Could you check a few things on this model? Use its own coordinates, in mm. Face numbers are marked on the shaded views. A direction names the side the tool comes from. Give positions to 0.01 mm unless a question says otherwise; leave off trailing zeros. Order: outer loops, then holes, each group sorted by start corner. A loop starts at its lowest first (then second) coordinate and runs counter-clockwise, first axis right, second up. Notation, with made-up numbers: M 13,8.25 L 31,8.25 A22 cw 31,40.25 Z; hole C -17,28.25 d8. An arc over 180 degrees is marked long. Answer in a Markdown table with one row per item. Add a question column.
```python
from build123d import *

# Parameters (mm, degrees)
SKETCH1_W                  = 10
SKETCH1_H                  = 10
BOSS_EXTRUDE1_DEPTH        = 10
SKETCH1_3_W                = 10
SKETCH1_3_H                = 10
BOSS_EXTRUDE2_DEPTH        = 15
BOSS_EXTRUDE3_DEPTH        = 15
SKETCH3_W                  = 20
SKETCH3_H                  = 5
BOSS_EXTRUDE4_DEPTH        = 20
F_4_0_209_DIAMETER_HOLE1_D = 5.3086
SKETCH5_W                  = 193
SKETCH5_H                  = 25
BOSS_EXTRUDE5_DEPTH        = 10
F_4_0_209_DIAMETER_HOLE2_D = 5.3086


with BuildPart() as part:
    # Sketch1 → Boss-Extrude1 (new body)
    with BuildSketch(Plane(origin=(0, 0, 0), x_dir=(1, 0, 0), z_dir=(0, 1, 0))):
        with Locations((-71.5, -38)):
            Rectangle(SKETCH1_W, SKETCH1_H)
        with Locations((-71.5, -48)):
            Rectangle(SKETCH1_W, SKETCH1_H)
        with Locations((-61.5, -48)):
            Rectangle(SKETCH1_W, SKETCH1_H)
        with Locations((-71.5, 38)):
            Rectangle(SKETCH1_W, SKETCH1_H)
        with Locations((-71.5, 48)):
            Rectangle(SKETCH1_W, SKETCH1_H)
        with Locations((-61.5, 48)):
            Rectangle(SKETCH1_W, SKETCH1_H)
        with Locations((61.5, 48)):
            Rectangle(SKETCH1_W, SKETCH1_H)
        with Locations((71.5, 48)):
            Rectangle(SKETCH1_W, SKETCH1_H)
        with Locations((71.5, 38)):
            Rectangle(SKETCH1_W, SKETCH1_H)
        with Locations((61.5, -48)):
            Rectangle(SKETCH1_W, SKETCH1_H)
        with Locations((71.5, -48)):
            Rectangle(SKETCH1_W, SKETCH1_H)
        with Locations((71.5, -38)):
            Rectangle(SKETCH1_W, SKETCH1_H)
    extrude(amount=BOSS_EXTRUDE1_DEPTH)

    # Sketch1_3 → Boss-Extrude2 (add)
    with BuildSketch(Plane(origin=(0, 0, 0), x_dir=(1, 0, 0), z_dir=(0, 1, 0))):
        with Locations((-71.5, -48)):
            Rectangle(SKETCH1_3_W, SKETCH1_3_H)
        with Locations((-61.5, -38)):
            Rectangle(SKETCH1_3_W, SKETCH1_3_H)
        with Locations((-61.5, -48)):
            Rectangle(SKETCH1_3_W, SKETCH1_3_H)
        with Locations((-71.5, -38)):
            Rectangle(SKETCH1_3_W, SKETCH1_3_H)
        with Locations((71.5, -48)):
            Rectangle(SKETCH1_3_W, SKETCH1_3_H)
        with Locations((71.5, -38)):
            Rectangle(SKETCH1_3_W, SKETCH1_3_H)
        with Locations((61.5, -48)):
            Rectangle(SKETCH1_3_W, SKETCH1_3_H)
        with Locations((61.5, -38)):
            Rectangle(SKETCH1_3_W, SKETCH1_3_H)
        with Locations((71.5, 38)):
            Rectangle(SKETCH1_3_W, SKETCH1_3_H)
        with Locations((71.5, 48)):
            Rectangle(SKETCH1_3_W, SKETCH1_3_H)
        with Locations((61.5, 48)):
            Rectangle(SKETCH1_3_W, SKETCH1_3_H)
        with Locations((61.5, 38)):
            Rectangle(SKETCH1_3_W, SKETCH1_3_H)
        with Locations((-61.5, 48)):
            Rectangle(SKETCH1_3_W, SKETCH1_3_H)
        with Locations((-61.5, 38)):
            Rectangle(SKETCH1_3_W, SKETCH1_3_H)
        with Locations((-71.5, 38)):
            Rectangle(SKETCH1_3_W, SKETCH1_3_H)
        with Locations((-71.5, 48)):
            Rectangle(SKETCH1_3_W, SKETCH1_3_H)
    extrude(amount=-BOSS_EXTRUDE2_DEPTH)

    # Sketch2 → Boss-Extrude3 (add)
    with BuildSketch(Plane(origin=(0, 0, 0), x_dir=(1, 0, 0), z_dir=(0, 1, 0))):
        Polygon((-59.664368284, 52.338863371), (-72.335631716, 32.661136629), (-21.409556012, -0.132169696), (0.205251763, 13.786456523), align=None)
        Polygon((0.205251763, 13.786456523), (-21.409556012, -0.132169696), (-0.205251763, -13.786456523), (21.409556012, 0.132169696), align=None)
        Polygon((59.784693164, 52.15200591), (0.205251763, 13.786456523), (21.409556012, 0.132169696), (72.215306836, 32.84799409), align=None)
        Polygon((21.409556012, 0.132169696), (-0.205251763, -13.786456523), (59.664368284, -52.338863371), (72.335631716, -32.661136629), align=None)
        Polygon((-0.205251763, -13.786456523), (-21.409556012, -0.132169696), (-72.215306836, -32.84799409), (-59.784693164, -52.15200591), align=None)
    extrude(amount=-BOSS_EXTRUDE3_DEPTH)

    # Sketch3 → Boss-Extrude4 (add)
    with BuildSketch(Plane.ZY.offset(76.5)):
        with Locations((-43, 7.5)):
            Rectangle(SKETCH3_W, SKETCH3_H)
        with Locations((43, 7.5)):
            Rectangle(SKETCH3_W, SKETCH3_H)
    boss_extrude4 = extrude(amount=BOSS_EXTRUDE4_DEPTH)

    # Mirror1: Boss-Extrude4 across plane
    add(boss_extrude4.mirror(Plane(origin=(0, 0, 0), x_dir=(0, 0, 1), z_dir=(1, 0, 0))))

    # 4 _0.209_ Diameter Hole1 (through all)
    with Locations(Plane(origin=(-86, 10, -42.5), x_dir=(0, 0, 1), z_dir=(0, 1, 0))):
        with Locations((0, 0), (85, 0), (0, 172), (85, 172)):
            Hole(F_4_0_209_DIAMETER_HOLE1_D / 2)

    # Sketch5 → Boss-Extrude5 (add)
    with BuildSketch(Plane.XY.offset(53)):
        with Locations((0, -2.5)):
            Rectangle(SKETCH5_W, SKETCH5_H)
    extrude(amount=BOSS_EXTRUDE5_DEPTH)

    # 4 _0.209_ Diameter Hole2 (through all)
    with Locations(Plane(origin=(0, 0, 53), x_dir=(-1, 0, 0), z_dir=(0, 0, -1))):
        with Locations((-86.5, -2.674811851), (86.5, -2.5)):
            Hole(F_4_0_209_DIAMETER_HOLE2_D / 2)


solid = part.part
```
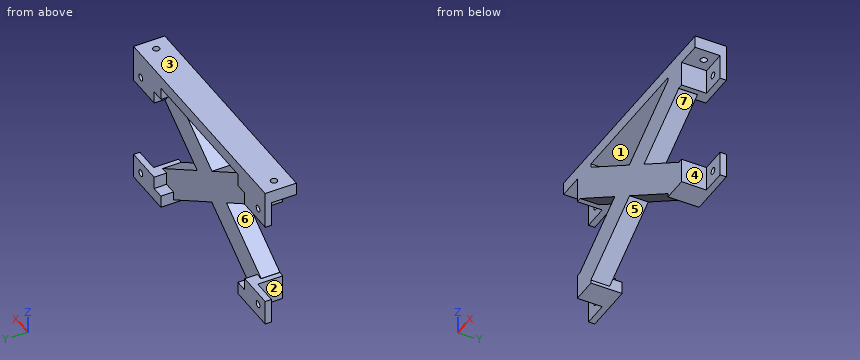
1. Will these pins go through, and if not, where does the flat tip stop? P1, Ø8.5, axis at x = -86, z = 42.5, coming from the -Y side; P2, Ø2, axis at y = -9.5, z = 17, coming from the +X side; P3, Ø10, axis at y = -12, z = 36.5, coming from the -X side.
2. Suppose I cut it at D-D on z = 9. List the corners of the cut face in (x, y) for me.
3. Suppose I cut it at B-B on x = 9. List the corners of the cut face in (y, z) for me, plus the area to 3 significant figures.
4. For the marked faces 4, 5, 6 and 7, which set-ups out of +Z, -Z, +X, -X, +Y, -Y let a thin tool reach every point of the face, with its end or its side?
5. Thinking about a two-plate mould opening in Z: for the marked faces 1, 2 and 3, which applies, pulls with the +Z half, pulls with the -Z half, needs draft (parallel to the pull), parting line crosses it, or undercut?
6. Suppose I cut it at C-C on x = 86. List the corners of the cut face in (y, z) for me.
7. If I drill on line 1 along X through (y, z) = (6.15, -42.5); line 2 along Z through (x, y) = (-31.5, -11.75); line 3 along Z through (x, y) = (-45.5, -6.5), over which ranges is the centre line in solid material (lowest first)? Write a range as [from, to].
Findings below:
| question | item | result |
|---|---|---|
| 1 | P1 | y = 5 |
| 1 | P2 | x = 49.57 |
| 1 | P3 | x = -76.5 |
| 2 | outline | M -35.18,-15 L 35.59,-15 L 35.59,0 L -35.18,0 Z |
| 3 | outline | M -15,-19.45 L 0,-19.45 L 0,19.71 L -15,19.71 Z; M -15,53 L 10,53 L 10,63 L -15,63 Z |
| 3 | area | 837 mm2 |
| 4 | face 4 | -Z, +X, -Y |
| 4 | face 5 | -Z, +Y, -Y |
| 4 | face 6 | -X, +Y, -Y |
| 4 | face 7 | +X, +Y, -Y |
| 5 | face 1 | undercut |
| 5 | face 2 | needs draft |
| 5 | face 3 | pulls with the +Z half |
| 6 | outline | M -15,53 L -5.28,53 L -5.28,63 L -15,63 Z; M -0.07,53 L 5,53 L 5,45.15 L 10,45.15 L 10,63 L -0.07,63 Z; M 5,-53 L 10,-53 L 10,-45.15 L 5,-45.15 Z; M 5,-39.85 L 10,-39.85 L 10,-33 L 5,-33 Z; M 5,33 L 10,33 L 10,39.85 L 5,39.85 Z |
| 7 | line 1 | [-96.5, -88.65], [-83.35, -66.5], [66.5, 83.35], [88.65, 96.5] |
| 7 | line 2 | [-34.2, -6.37], [6.63, 33.94], [53, 63] |
| 7 | line 3 | [-43.22, -15.38], [15.64, 42.95], [53, 63] |
